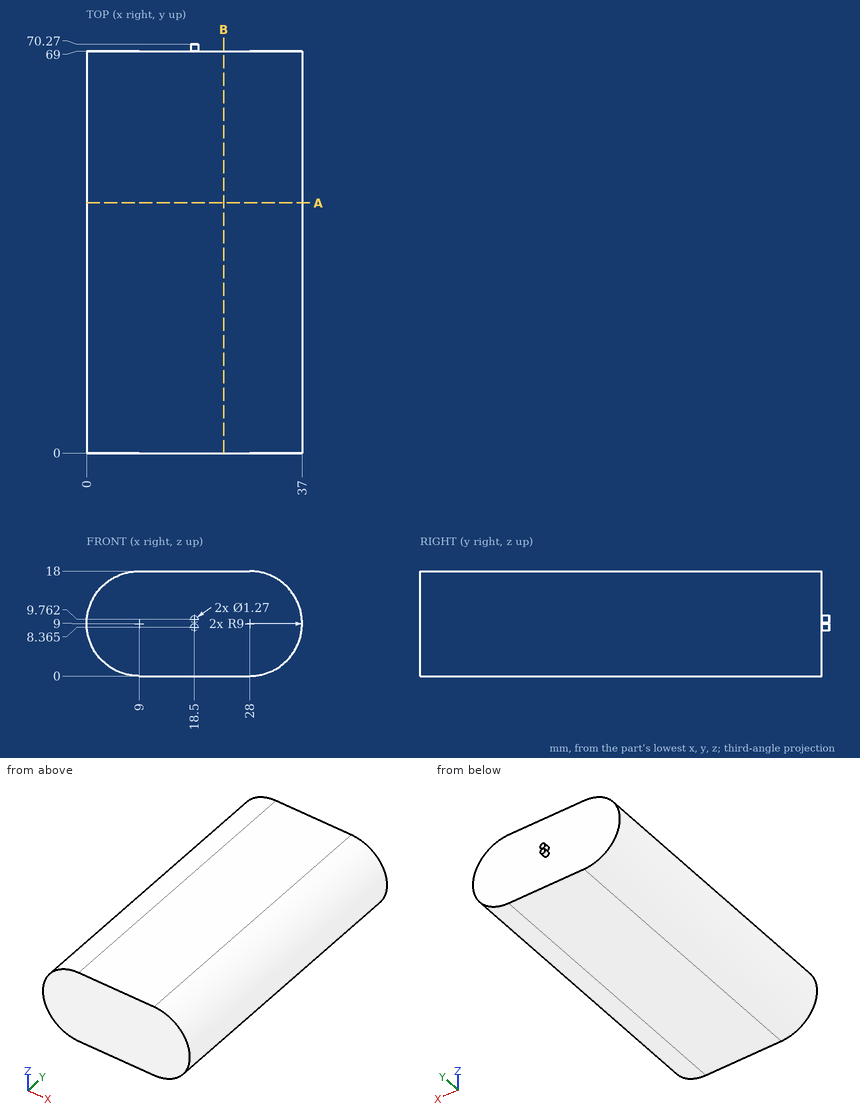
Input: dimensioned drawing with shaded views. Units: mm. Origin: part minimum x, y, z. Give positions to 0.01 mm unless a question says otherwise; leave off trailing zeros. Write each loop counter-clockwise with the first axis right and the second up, starting at its lowest first coordinate (ties: lowest second). Pieces come first, ordered by that corner, then holes. Notation, with made-up numbers: M 5.5,-14.5 L 9.5,-14.5 A22 ccw 9.5,2.5 Z; hole C 53.25,74 d8. An arc over 180 degrees is marked long. Return JSON: item names as keys, results as strings. Group by question number.
1) Material intervals for line 1 along Y through (x, z) = (9.5, 5); line 2 along Z through (x, y) = (8.5, 52); line 3 along X through (y, z) = (7.5, 12.5), sorted ascending. Write a range as [from, to].
2) Pin query (flat end, axial travel): P1, Ø1.5, axis at y = 60, z = 4, coming from the -X side; P2, Ø1.5, axis at y = 54, z = 7, coming from the -X side; P3, Ø1, axis at x = 20.5, z = 5, coming from the +Y side. Return the tip coordinate at first contact, or that it passes through.
3) Cut plane A-A, the plane y = 43. Output: boundary loops of the cut face in (x, z), plus the area to 3 significant figures.
4) Cut plane B-B, the plane x = 23.5. Output: boundary loops of the cut face in (y, z), plus the area to 3 significant figures.
Recorded:
{
 "1": {"line 1": "y = [0, 69]", "line 2": "z = [0.01, 17.99]", "line 3": "x = [0.71, 36.29]"},
 "2": {"P1": "stops at x = 1.07", "P2": "stops at x = 0.09", "P3": "stops at y = 69"},
 "3": {"outline": "M 9,0 L 28,0 A9 ccw 28,18 L 9,18 A9 ccw Z", "area": "596 mm²"},
 "4": {"outline": "M 0,0 L 69,0 L 69,18 L 0,18 Z", "area": "1,240 mm²"}
}
